```python
from build123d import *

# Parameters (mm, degrees)
F1_ANGLE  = 180
F3_DEPTH  = 10
F4_R      = 15.9
F5_DEPTH  = 12.5
F6_R      = 2.4
F7_DEPTH  = 8.211553
F9_DEPTH  = 1.2
F11_DEPTH = 1.2


with BuildPart() as f1:
    # F0 (on Front) → F1 (revolve, symmetric)
    with BuildSketch(Plane.XZ) as f1_sk:
        Polygon((-5.9, 14.764823), (-2.4, 15.717824), (-2.4, 19.764823), (-3.9, 19.764823), (-3.9, 36.764823), (-2.4, 36.764823), (-2.4, 38.764823), (-5.9, 38.764823), align=None)
    revolve(axis=Axis((0, 0, 26.233703), (0, 0, 1)), revolution_arc=F1_ANGLE / 2)
    revolve(f1_sk.sketch, axis=Axis((0, 0, 26.233703), (0, 0, -1)), revolution_arc=F1_ANGLE / 2)

    # F2 (on Front) → F3 (join, symmetric)
    with BuildSketch(Plane.XZ):
        with BuildLine():
            ThreePointArc((-10.922859, 11.55427), (-5.877802, 14.773674), (0, 15.9))
            Line((0, 15.9), (0, 18))
            ThreePointArc((0, 18), (-6.432893, 16.811243), (-12.016103, 13.401987))
            Line((-12.016103, 13.401987), (-10.922859, 11.55427))
        make_face()
    extrude(amount=F3_DEPTH, both=True)

    # F4 (on Front) → F5 (cut, symmetric)
    with BuildSketch(Plane.XZ):
        Circle(F4_R)
    extrude(amount=F5_DEPTH, both=True, mode=Mode.SUBTRACT)

    # F6 (on face) → F7 (cut, through all)
    with BuildSketch(Plane.XY.offset(19.764823)):
        Circle(F6_R)
    extrude(amount=-F7_DEPTH, mode=Mode.SUBTRACT)

    # F8 (on face) → F9 (join)
    with BuildSketch(Plane.XZ.offset(10)):
        with BuildLine():
            ThreePointArc((-10.922859, 11.55427), (-5.877802, 14.773674), (0, 15.9))
            Line((0, 15.9), (0, 19.290676))
            ThreePointArc((0, 19.290676), (-5.655412, 18.443061), (-10.813836, 15.974703))
            Line((-10.813836, 15.974703), (-10.922859, 11.55427))
        make_face()
    extrude(amount=F9_DEPTH)

    # F10 (on face) → F11 (join)
    with BuildSketch(Plane(origin=(0, 10, 0), x_dir=(-1, 0, 0), z_dir=(0, 1, 0))):
        with BuildLine():
            Line((0, 19.332207), (0, 15.9))
            ThreePointArc((0, 15.9), (5.877802, 14.773674), (10.922859, 11.55427))
            Line((10.922859, 11.55427), (10.814505, 16.024379))
            ThreePointArc((10.814505, 16.024379), (5.654539, 18.486764), (0, 19.332207))
        make_face()
    extrude(amount=F11_DEPTH)


solid = f1.part
```
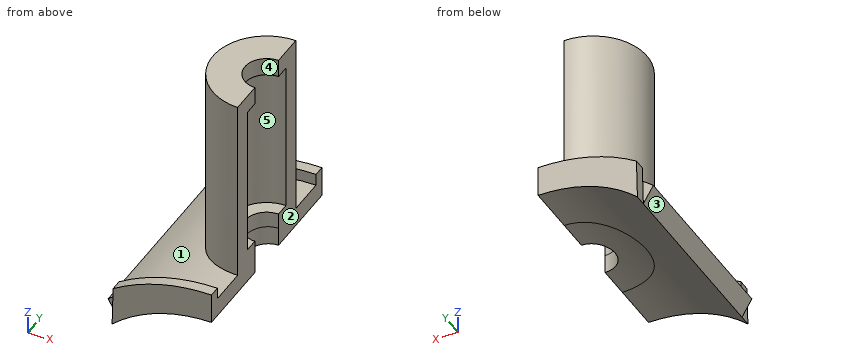
Part model, mm, in its own coordinate system. Face numbers are marked on the shaded views. A direction names the side the tool comes from. Round coordinates to 2 decimals unless told otherwise and drop trailing zeros. Loops run counter-clockwise (first coordinate to the right, second up) from the corner with the lowest first, then second, coordinate; pieces in that order, holes last. Notation, with made-up numbers: (16.5, 44) -> (60.5, 44) arc R20 ccw to (60.5, 65) -> close; hole circle Ø7 at (27, 3.5). An arc over 180 degrees is marked (long way). Use one line per item in the form item = value. Start each with the question number.
Item 1: Drill centre lines: line 1 along Y through (x, z) = (-4, 18); line 2 along Z through (x, y) = (-0.5, 10.5); line 3 along Z through (x, y) = (-2.25, -3). Where is each one in solid material? Low to high.
Item 2: Band-saw the part on B-B (x = -7.25). List the corners of the cut face in (y, z), plus the area to 3 significant figures.
Item 3: Band-saw the part on D-D (x = -3). List the corners of the cut face in (y, z).
Item 4: Band-saw the part on C-C (z = 30). List the corners of the cut face in (x, y), plus the area to 3 significant figures.
Item 5: Two-plate mould, pull along Z, no slides. Class the marked faces 3, 4 and 5: released by +Z, released by -Z, zero draft, split by the parting line, or undercut.
Item 6: Band-saw the part on A-A (y = 0). List the corners of the cut face in (x, z).
Item 7: Tool access for the marked faces 1 and 2: list every direction of +Z, -Z, +X, -X, +Y, -Y with a clear straight run to the whole face (end or side of a thin tool).
Item 8: Drop flat-ended pins along their axis: pin 1 Ø0.6 at (x, z) = (-11.5, 13) entering from -Y; pin 2 Ø1.5 at (x, y) = (-1.5, 0.5) entering from +Z; pin 3 Ø1.5 at (x, y) = (-10.5, -6) entering from +Z; pin 4 Ø12 at (y, z) = (-2, 33.5) entering from -X. Give the stop position or say it passes through.
Data:
q1.line_1 = -11.2 to -10, -4.34 to 4.34, 10 to 11.2
q1.line_2 = 15.89 to 19.33
q1.line_3 = 15.74 to 19.76, 36.76 to 38.76
q2.outline = (-11.2, 14.15) -> (11.2, 14.15) -> (11.2, 17.92) -> (10, 17.92) -> (10, 16.48) -> (-10, 16.48) -> (-10, 17.88) -> (-11.2, 17.88) -> close
q2.area = 55.5 mm^2
q3.outline = (-11.2, 15.61) -> (11.2, 15.61) -> (11.2, 19.1) -> (10, 19.1) -> (10, 17.75) -> (5.08, 17.75) -> (5.08, 38.76) -> (-5.08, 38.76) -> (-5.08, 17.75) -> (-10, 17.75) -> (-10, 19.06) -> (-11.2, 19.06) -> close; hole (-2.49, 19.76) -> (2.49, 19.76) -> (2.49, 36.76) -> (-2.49, 36.76) -> close
q4.outline = (0, -5.9) -> (0, -3.9) arc R3.9 cw to (0, 3.9) -> (0, 5.9) arc R5.9 ccw to start
q4.area = 30.8 mm^2
q5.face_3 = released by -Z
q5.face_4 = zero draft
q5.face_5 = undercut
q6.outline = (-12.02, 13.4) -> (-10.92, 11.55) arc R15.9 cw to (-2.4, 15.72) -> (-2.4, 19.76) -> (-3.9, 19.76) -> (-3.9, 36.76) -> (-2.4, 36.76) -> (-2.4, 38.76) -> (-5.9, 38.76) -> (-5.9, 17.01) arc R18 ccw to start
q7.face_1 = +Z, -X
q7.face_2 = +Z, -Z, +X, +Y, -Y
q8.pin_1 = -10
q8.pin_2 = through
q8.pin_3 = 15.13
q8.pin_4 = -5.9
